For this review, take the finished solid that the model builds, in its own axes (mm). Face numbers are marked on the shaded views. A direction names the side the tool comes from. Coordinates: 2 decimals unless noted, no trailing zeros. Order: outer loops, then holes, each group sorted by start corner. A loop starts at its lowest first (then second) coordinate and runs counter-clockwise, first axis right, second up. Notation, with made-up numbers: (-6, 9.25) -> (37, 9.25) arc R31 cw to (37, 47.25) -> close; hole circle Ø7 at (-16.5, -12.5). An arc over 180 degrees is marked (long way). Write item = value, one per line. Start each with the question number.
1) Consider section B-B on y = 61. Give the boundary of the cut face in (x, z), and give its area (3 significant figures).
2) Wall thickness on probe 1 along Z at (x, y) = (-4, 56.5); probe 2 along Y at (x, z) = (-46, -81.5): over which ranges is each line inside the solid? List them lowest first. Write a range as [from, to].
3) Consider section A-A on x = -45. Give the boundary of the cut face in (y, z).
4) Insertion check: pin 1 Ø5 at (x, y) = (-38.5, 54.5) entering from +Z; pin 2 Ø5 at (x, y) = (-30, 59) entering from -Z; pin 3 Ø2 at (x, z) = (-38, -69.5) entering from +Y. Each pin has a flat end and moves straight along its axis. Give the tip position at first contact, or say it passes through.
5) Machinability: for the marked faces 1, 2 and 3, which of the approach directions +Z, -Z, +X, -X, +Y, -Y give a long, thin tool a straight path to every point of the face, cutting with its end or side? Answer none if there is none.
Autodesk Inventor part; units mm, degrees
ref_plane "YZ Plane" through (0, 0, 0) normal (1, 0, 0) x (0, 1, 0)
ref_plane "XZ Plane" through (0, 0, 0) normal (0, 1, 0) x (-1, 0, 0)
ref_plane "XY Plane" through (0, 0, 0) normal (0, 0, 1) x (1, 0, 0)
sketch "Sketch1" plane through (0, 0, 0) normal (0, 1, 0) x (-1, 0, 0)
  line L0 (0, 0) -> (50.8, 0)
  line L1 (50.8, 0) -> (50.8, -400)
  line L2 (50.8, -400) -> (0, -400)
  line L3 (0, -400) -> (0, 0)
  dimension "d0" = 50.8
  dimension "d1" = 400
extrude "Extrusion1" add sketch "Sketch1" along normal blind 77
sketch "Sketch3" plane through (0, 0, 0) normal (1, 0, 0) x (0, 0, -1)
  line L0 (0, 77) -> (101.6, 77)
  line L1 (101.6, 77) -> (101.6, 51.2)
  line L2 (101.6, 51.2) -> (0, 51.2)
  line L3 (0, 51.2) -> (0, 77)
  line L4 (0, 77) -> (400, 77)
  line L5 (400, 77) -> (285, 77)
  line L6 (285, 77) -> (285, 51.2)
  line L7 (285, 51.2) -> (400, 51.2)
  line L8 (400, 51.2) -> (400, 77)
  point P0 (0, 0)
  dimension "d8" = 101.6
  dimension "d9" = 25.8
  dimension "d10" = 115
  dimension "d11" = 25.8
extrude "Extrusion2" cut sketch "Sketch3" against normal blind 50.8
properties part number "PiezaPuerta-1"
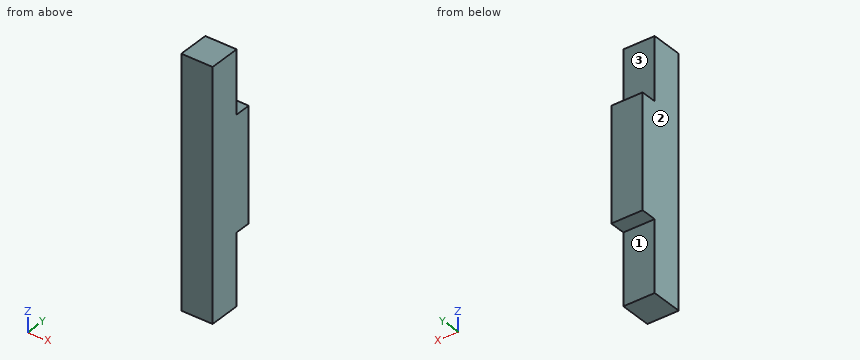
Answer sheet:
q1.outline = (-50.8, -285) -> (0, -285) -> (0, -101.6) -> (-50.8, -101.6) -> close
q1.area = 9,320 mm2
q2.probe_1 = [-285, -101.6]
q2.probe_2 = [0, 51.2]
q3.outline = (0, -400) -> (51.2, -400) -> (51.2, -285) -> (77, -285) -> (77, -101.6) -> (51.2, -101.6) -> (51.2, 0) -> (0, 0) -> close
q4.pin_1 = -101.6
q4.pin_2 = -285
q4.pin_3 = 51.2
q5.face_1 = -Z, +X, -X, +Y
q5.face_2 = +Z, -Z, -X, +Y, -Y
q5.face_3 = +Z, +X, -X, +Y
